```python
from build123d import *

# Parameters (mm, degrees)
SKETCH1_W                   = 65
SKETCH1_H                   = 52
BASE_EXTRUDE_DEPTH          = 7.5
F_1_4_20_TAPPED_HOLE1_D     = 5.1054
F_1_4_20_TAPPED_HOLE1_DEPTH = 16.51
F_1_4_20_TAPPED_HOLE1_TIP   = 1.533816902
F_1_4_CLEARANCE_HOLE1_D     = 6.7564
F_8_32_TAPPED_HOLE1_D       = 3.4544
CUT_EXTRUDE1_REACH          = 17
SKETCH8_R                   = 0.508


with BuildPart() as part:
    # Sketch1 → Base-Extrude (new body, symmetric)
    with BuildSketch(Plane.XY):
        Rectangle(SKETCH1_W, SKETCH1_H)
    extrude(amount=BASE_EXTRUDE_DEPTH, both=True)

    # 1/4-20 Tapped Hole1
    with Locations(Plane(origin=(0, 26, 0), x_dir=(-1, 0, 0), z_dir=(0, 1, 0))):
        with Locations((5, 0), (-10, 0)):
            Hole(F_1_4_20_TAPPED_HOLE1_D / 2, depth=F_1_4_20_TAPPED_HOLE1_DEPTH)
            with Locations((0, 0, -(F_1_4_20_TAPPED_HOLE1_DEPTH + F_1_4_20_TAPPED_HOLE1_TIP / 2))):  # 118° drill point
                Cone(0, F_1_4_20_TAPPED_HOLE1_D / 2, F_1_4_20_TAPPED_HOLE1_TIP, mode=Mode.SUBTRACT)

    # 1/4 Clearance Hole1 (through all)
    with Locations(Plane(origin=(0, 26, 0), x_dir=(-1, 0, 0), z_dir=(0, 1, 0))):
        with Locations((-25, 0), (25, 0)):
            Hole(F_1_4_CLEARANCE_HOLE1_D / 2)

    # #8-32 Tapped Hole1 (through all)
    with Locations(Plane(origin=(0, 0, -7.5), x_dir=(-1, 0, 0), z_dir=(0, 0, -1))):
        with Locations((-2.5, 2.7)):
            Hole(F_8_32_TAPPED_HOLE1_D / 2)

    # Sketch8 → Cut-Extrude1 (cut, up to next)
    with BuildSketch(Plane.XY.offset(7.5), mode=Mode.PRIVATE) as cut_extrude1_sk1:
        with Locations((10, 13.3)):
            Circle(SKETCH8_R)
    cut_extrude1_tool1 = extrude(cut_extrude1_sk1.sketch, amount=-CUT_EXTRUDE1_REACH, mode=Mode.PRIVATE) & part.part
    add(cut_extrude1_tool1.solids().sort_by_distance((10, 13.3, 7.5))[0], mode=Mode.SUBTRACT)
    # Sketch8 → Cut-Extrude1 (cut, up to next)
    with BuildSketch(Plane.XY.offset(7.5), mode=Mode.PRIVATE) as cut_extrude1_sk2:
        with Locations((-5, 13.3)):
            Circle(SKETCH8_R)
    cut_extrude1_tool2 = extrude(cut_extrude1_sk2.sketch, amount=-CUT_EXTRUDE1_REACH, mode=Mode.PRIVATE) & part.part
    add(cut_extrude1_tool2.solids().sort_by_distance((-5, 13.3, 7.5))[0], mode=Mode.SUBTRACT)


solid = part.part
```
The model under review builds one solid part; all positions refer to its coordinate system, in mm. A direction names the side the tool comes from. Round coordinates to 2 decimals unless told otherwise and drop trailing zeros. Loops run counter-clockwise (first coordinate to the right, second up) from the corner with the lowest first, then second, coordinate; pieces in that order, holes last. Notation, with made-up numbers: (37.5, 39) -> (85.5, 39) arc R25 ccw to (85.5, 59) -> close; hole circle Ø7 at (24.5, 10.5). An arc over 180 degrees is marked (long way). Answer in a Markdown table with one row per item.
1) Tool access review of faces 1 (the cylindrical face through (12.435, 17.629, 0.767)), 2 (the flat face through (-32.5, 0, 0)): name each direction out of +Z, -Z, +X, -X, +Y, -Y from which nothing blocks a thin tool from reaching the whole face with its end or side.
Taken from the geometry:
| item | result |
|---|---|
| face 1 | +Y |
| face 2 | +Z, -Z, -X, +Y, -Y |
2) Wall thickness on line 1 along X through (y, z) = (13.3, 4.15); line 2 along Z through (x, y) = (-25, 11); line 3 along Z through (x, y) = (-5, 17): over which ranges is each line inside the solid? List them lowest first.
Taken from the geometry:
| item | result |
|---|---|
| line 1 | x = -32.5 to -5.51, -4.49 to 9.49, 10.51 to 32.5 |
| line 2 | z = -7.5 to -3.38, 3.38 to 7.5 |
| line 3 | z = -7.5 to -2.55, 2.55 to 7.5 |
3) Consider section B-B, the plane x = 2.5. Write out the cut boundary in (y, z).
Taken from the geometry:
| item | result |
|---|---|
| outline | (-26, -7.5) -> (0.97, -7.5) -> (0.97, 7.5) -> (-26, 7.5) -> close; (4.43, -7.5) -> (26, -7.5) -> (26, 7.5) -> (4.43, 7.5) -> close |
4) Consider section A-A, the plane y = 2.7. Write out the cut boundary in (x, z), plus the area to 3 significant figures.
Taken from the geometry:
| item | result |
|---|---|
| outline | (-32.5, -7.5) -> (0.77, -7.5) -> (0.77, 7.5) -> (-32.5, 7.5) -> close; (4.23, -7.5) -> (32.5, -7.5) -> (32.5, 7.5) -> (4.23, 7.5) -> close; hole circle Ø6.76 at (-25, 0); hole circle Ø6.76 at (25, 0) |
| area | 851 mm² |
5) Consider section C-C, the plane y = 16. Write out the cut boundary in (x, z), plus the area to 3 significant figures.
Taken from the geometry:
| item | result |
|---|---|
| outline | (-32.5, -7.5) -> (32.5, -7.5) -> (32.5, 7.5) -> (-32.5, 7.5) -> close; hole circle Ø6.76 at (-25, 0); hole circle Ø5.11 at (-5, 0); hole circle Ø5.11 at (10, 0); hole circle Ø6.76 at (25, 0) |
| area | 862 mm² |
6) Consider section D-D, the plane y = -16. Write out the cut boundary in (x, z).
Taken from the geometry:
| item | result |
|---|---|
| outline | (-32.5, -7.5) -> (32.5, -7.5) -> (32.5, 7.5) -> (-32.5, 7.5) -> close; hole circle Ø6.76 at (-25, 0); hole circle Ø6.76 at (25, 0) |
7) Draft analysis for pull direction Z (two halves, no side actions). For faces 3 (the cylindrical face through (3.3, 1.17, 0.11)), 4 (the flat face through (0, 0, 7.5)), 5 (the flat face through (0, 0, -7.5)), 6 (the conical face through (-4.673, 8.223, 0.3)), state which applies: pulls with the +Z half, pulls with the -Z half, needs draft (parallel to the pull), parting line crosses it, or undercut.
Taken from the geometry:
| item | result |
|---|---|
| face 3 | needs draft |
| face 4 | pulls with the +Z half |
| face 5 | pulls with the -Z half |
| face 6 | undercut |
